Input: part model. Units: mm. Frame: model coordinates. Face numbers are marked on the shaded views. A direction names the side the tool comes from. Give positions to 0.01 mm unless a question says otherwise; leave off trailing zeros. Loops run counter-clockwise (first coordinate to the right, second up) from the corner with the lowest first, then second, coordinate; pieces in that order, holes last. Notation, with made-up numbers: (-25, 51) -> (25, 51) arc R21 ccw to (25, 55) -> close; hole circle Ø10 at (71.25, -22). An arc over 180 degrees is marked (long way). Use CSV: the item, a comma, the result in double quotes.
```python
from build123d import *

# Parameters (mm, degrees)
F0_W     = 96.52
F0_H     = 96.52
F1_DEPTH = 6.35
F2_W     = 96.52
F2_H     = 96.52
F2_W_2   = 88.9
F2_H_2   = 88.9
F3_DEPTH = 16.51
F4_R     = 6.35
F5_DEPTH = 6.351


with BuildPart() as f1:
    # F0 (on Top) → F1 (new body)
    with BuildSketch(Plane.XY):
        with Locations((48.26, 48.26)):
            Rectangle(F0_W, F0_H)
    extrude(amount=F1_DEPTH)

    # F2 (on face) → F3 (join)
    with BuildSketch(Plane.XY.offset(6.35)):
        with Locations((48.26, 48.26)):
            Rectangle(F2_W, F2_H)
        with Locations((48.26, 48.26)):
            Rectangle(F2_W_2, F2_H_2, mode=Mode.SUBTRACT)
    extrude(amount=F3_DEPTH)

    # F4 (on face) → F5 (cut, through all)
    with BuildSketch(Plane.XY.offset(6.35)):
        with Locations((19.974461, 76.545539)):
            Circle(F4_R)
        with Locations((19.974461, 19.974461)):
            Circle(F4_R)
        with Locations((76.545539, 19.974461)):
            Circle(F4_R)
        with Locations((76.545539, 76.545539)):
            Circle(F4_R)
    extrude(amount=-F5_DEPTH, mode=Mode.SUBTRACT)


solid = f1.part
```
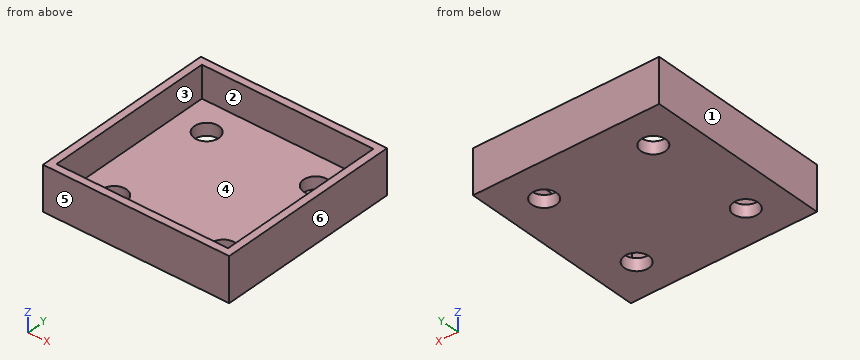
1) Section query C-C (y = 22.5). Return loops of the section in (x, z), then the cut area to 3 significant figures.
From the geometry:
outline,"(0, 0) -> (14.15, 0) -> (14.15, 6.35) -> (3.81, 6.35) -> (3.81, 22.86) -> (0, 22.86) -> close; (25.8, 0) -> (70.72, 0) -> (70.72, 6.35) -> (25.8, 6.35) -> close; (82.37, 0) -> (96.52, 0) -> (96.52, 22.86) -> (92.71, 22.86) -> (92.71, 6.35) -> (82.37, 6.35) -> close"
area,"591 mm^2"
2) Mould query, pull axis X, two halves, no side actions, for the marked faces 3, 4, 5 and 6. Classes: pulls with the +X half, pulls with the -X half, needs draft (parallel to the pull), parting line crosses it, or undercut.
From the geometry:
face 3,"undercut"
face 4,"undercut"
face 5,"needs draft"
face 6,"pulls with the +X half"
3) Ray query, line 1 (Y direction, x = 37, z = 7); line 2 (Z direction, x = 68, y = 5). Return the intervals inside material, ascending.
From the geometry:
line 1,"y = 0 to 3.81, 92.71 to 96.52"
line 2,"z = 0 to 6.35"
4) Contact query for a flat-ended pin moving along its axis: pin 1 (1.5 mm diameter, centred on x = 62.5, y = 76, fed in from +Z). Output: stop coordinate, or through.
From the geometry:
pin 1,"stops at z = 6.35"
5) Reachability of the marked faces 1 and 2 from +Z, -Z, +X, -X, +Y, -Y: full face, straight path, thin tool, end or side. Return the list, or none.
From the geometry:
face 1,"+Z, -Z, -X, +Y, -Y"
face 2,"+Z"
6) Section query B-B (x = 62). Return loops of the section in (y, z).
From the geometry:
outline,"(0, 0) -> (96.52, 0) -> (96.52, 22.86) -> (92.71, 22.86) -> (92.71, 6.35) -> (3.81, 6.35) -> (3.81, 22.86) -> (0, 22.86) -> close"
7) Section query D-D (x = 20). Return loops of the section in (y, z), then the cut area to 3 significant figures.
From the geometry:
outline,"(0, 0) -> (13.62, 0) -> (13.62, 6.35) -> (3.81, 6.35) -> (3.81, 22.86) -> (0, 22.86) -> close; (26.32, 0) -> (70.2, 0) -> (70.2, 6.35) -> (26.32, 6.35) -> close; (82.9, 0) -> (96.52, 0) -> (96.52, 22.86) -> (92.71, 22.86) -> (92.71, 6.35) -> (82.9, 6.35) -> close"
area,"577 mm^2"
8) Section query A-A (z = 10.5). Return loops of the section in (x, y), then the cut area to 3 significant figures.
From the geometry:
outline,"(0, 0) -> (96.52, 0) -> (96.52, 96.52) -> (0, 96.52) -> close; hole (3.81, 3.81) -> (92.71, 3.81) -> (92.71, 92.71) -> (3.81, 92.71) -> close"
area,"1,410 mm^2"
